Part model, mm, in its own coordinate system. A direction names the side the tool comes from. Give positions to 0.01 mm unless a question says otherwise; leave off trailing zeros. Write each loop counter-clockwise with the first axis right and the second up, starting at its lowest first coordinate (ties: lowest second). Pieces come first, ordered by that corner, then holes.
from build123d import *

# Parameters (mm, degrees)
CYLINDER032_R              = 1.7
CYLINDER032_DEPTH          = 20
EXTRUDE005_DEPTH           = 9
EXTRUDE005_PLACEMENT_ANGLE = 90
BOX044_W                   = 10
BOX044_H                   = 8
BOX044_DEPTH               = 8
CUT053_PLACEMENT_ANGLE     = 180
BOX043_W                   = 20
BOX043_H                   = 20
BOX043_DEPTH               = 3


with BuildPart() as cylinder032:
    # Cylinder032 → Cylinder032 (new body)
    with BuildSketch(Plane(origin=(140, 9.74, 51.5), x_dir=(0, 0, -1), z_dir=(1, 0, 0))):
        Circle(CYLINDER032_R)
    extrude(amount=CYLINDER032_DEPTH)


with BuildPart() as extrude005:
    # Sketch005 → Extrude005 (new body)
    with BuildSketch(Plane.XY.offset(75)):
        Polygon((-29.694611, 6.813304), (-28.00073, 9.738351), (-29.686954, 12.667818), (-33.06706, 12.672239), (-34.760941, 9.747192), (-33.074716, 6.817725), align=None)
    extrude(amount=EXTRUDE005_DEPTH)


with BuildPart() as extrude005_1:
    # Extrude005 placement: moved
    add(extrude005.part.moved(Location((71, 0, 0))).rotate(Axis((71, 0, 0), (0, 1, 0)), EXTRUDE005_PLACEMENT_ANGLE))


with BuildPart() as cut053:
    # Box044 → Box044 (new body)
    with BuildSketch(Plane(origin=(144, 5.745, 27.5), x_dir=(1, 0, 0), z_dir=(0, 0, 1))):
        with Locations((5, 4)):
            Rectangle(BOX044_W, BOX044_H)
    extrude(amount=BOX044_DEPTH)

    # Cut052: cut Extrude005
    add(extrude005_1.part, mode=Mode.SUBTRACT)


with BuildPart() as cut053_1:
    # Cut052 placement: moved
    add(cut053.part.moved(Location((0, 0, 20))))

    # Cut053: cut Cylinder032
    add(cylinder032.part, mode=Mode.SUBTRACT)


with BuildPart() as cut053_2:
    # Cut053 placement: moved
    add(cut053_1.part.moved(Location((398, 10, 103))).rotate(Axis((398, 10, 103), (0, 1, 0)), CUT053_PLACEMENT_ANGLE))


with BuildPart() as topmounttest:
    # Box043 → Box043 (new body)
    with BuildSketch(Plane(origin=(235.5, 10, 55.5), x_dir=(1, 0, 0), z_dir=(0, 0, 1))):
        with Locations((10, 10)):
            Rectangle(BOX043_W, BOX043_H)
    extrude(amount=BOX043_DEPTH)

    # Fusion002: union Cut053
    add(cut053_2.part)


solid = topmounttest.part
1) Mould opens along Z. For faces 5 (the flat face through (249, 20, 47.5)), 6 (the flat face through (248.06, 18.3, 49.07)), 7 (the flat face through (245, 20, 58.5)), 8 (the flat face through (254, 18.8, 49.8)) say: +Z half, -Z half, draft (parallel to the pull), parting line (faces both ways), or undercut.
Check result:
face 5: -Z half
face 6: undercut
face 7: +Z half
face 8: draft
2) Saw through at C-C (z = 54.25). Write the cut outline in (x, y) (3 decimals), and give its area (3 significant figures).
Check result:
outline: (244, 15.745) - (254, 15.745) - (254, 23.745) - (244, 23.745) - (244, 21.04) - (252, 21.04) - (252, 18.444) - (244, 18.444) - close
area: 59.2 mm2
3) Saw through at A-A (x = 252.25). Write the cut outline in (y, z) (3 decimals).
Check result:
outline: (10, 55.5) - (15.745, 55.5) - (15.745, 47.5) - (23.745, 47.5) - (23.745, 55.5) - (30, 55.5) - (30, 58.5) - (10, 58.5) - close; hole circle Ø3.4 at (19.74, 51.5)
4) 3-axis set-ups, long thin cutter, end or side, ignore diameter. For faces 1 (the flat face through (249, 23.745, 52)), 2 (the flat face through (248.056, 18.255, 54.14)), 3 (the flat face through (249, 15.745, 52)), 4 (the flat face through (244, 18, 49)): which of +Z, -Z, +X, -X, +Y, -Y reach the whole face in a straight line?
Check result:
face 1: -Z, +X, -X, +Y
face 2: -X
face 3: -Z, +X, -X, -Y
face 4: -Z, -X, +Y, -Y
5) Drill centre lines: L1, parallel to Y at x = 253.3, z = 51.5 (3 decimals); L2, parallel to Z at x = 244.75, y = 27.75; L3, parallel to X at y = 22, z = 55. Where is each one in solid material? Low to high.
Check result:
L1: y = 15.745 to 18.04, 21.44 to 23.745
L2: z = 55.5 to 58.5
L3: x = 244 to 254
6) Flat gauge pins, fed straight in: P1, Ø2.5, axis at x = 247, z = 51, coming from the -Y side (3 decimals); P2, Ø3, axis at y = 23, z = 52.5, coming from the -X side; P3, Ø3, axis at y = 19, z = 51, coming from the -X side. Where does each tip first touch, or does it go through?
Check result:
P1: stops at y = 15.745
P2: stops at x = 244
P3: stops at x = 252
7) Saw through at B-B (y = 16.25). Write the cut outline in (x, z), and give its area (3 significant figures).
Check result:
outline: (235.5, 55.5) - (244, 55.5) - (244, 47.5) - (254, 47.5) - (254, 55.5) - (255.5, 55.5) - (255.5, 58.5) - (235.5, 58.5) - close
area: 140 mm2
8) Saw through at D-D (z = 51.5). Write the cut outline in (x, y) (3 decimals).
Check result:
outline: (244, 15.745) - (254, 15.745) - (254, 18.04) - (252, 18.04) - (252, 16.816) - (244, 16.816) - close; (244, 22.67) - (252, 22.67) - (252, 21.44) - (254, 21.44) - (254, 23.745) - (244, 23.745) - close
